For this review, take the finished solid that the model builds, in its own axes (mm). A direction names the side the tool comes from. Coordinates: 2 decimals unless noted, no trailing zeros. Loops run counter-clockwise (first coordinate to the right, second up) from the corner with the lowest first, then second, coordinate; pieces in that order, holes last. Notation, with made-up numbers: M 35.5,85.25 L 41.5,85.25 A15 ccw 41.5,98.25 Z; hole C -32.5,65 d4. An arc over 180 degrees is marked long. Write each question's results on one line, items separated by ' | '. Start each with the question number.
```python
from build123d import *

# Parameters (mm, degrees)
EXTRUDE_1_DEPTH     = 20
SKETCH_2_R          = 2
CUT_EXTRUDE_1_DEPTH = 20


with BuildPart() as part:
    # 草图1 → 凸台-拉伸1 (new body)
    with BuildSketch(Plane.XY):
        Polygon((-17.175607408, 36.360314389), (-7.175607408, 36.360314389), (2.824392592, 36.360314389), (2.824392592, 34.360314389), (-17.175607408, 34.360314389), (-17.175607408, -0.639685611), (-17.175607408, -2.639685611), (-47.175607408, -2.639685611), (-47.175607408, -0.639685611), (-19.175607408, -0.639685611), (-19.175607408, 36.360314389), align=None)
    extrude(amount=EXTRUDE_1_DEPTH)

    # 草图2 → 切除-拉伸1 (cut)
    with BuildSketch(Plane(origin=(0, 36.360314389, 0), x_dir=(1, 0, 0), z_dir=(0, 1, 0))):
        with Locations((-2.175607408, -10)):
            Circle(SKETCH_2_R)
    extrude(amount=-CUT_EXTRUDE_1_DEPTH, mode=Mode.SUBTRACT)


solid = part.part
```
Q1. For faces 4 (the face through (-19.176, 18, 10)), 5 (the face through (-7, 34.36, 10)), 6 (the face through (-8, 36.36, 10)), list the 3-axis set-ups (+Z, -Z, +X, -X, +Y, -Y) from which the entire face can be reached by the end or side of a thin tool; tool diameter is ignored.
Q2. To check wall thickness, follow line 1 along X through (y, z) = (35.65, 10); line 2 along Y through (x, z) = (-33, 15.5); line 3 along X through (y, z) = (18.5, 15). State the ranges of each line that lie inside material, in increasing order.
Q3. Take a section at B-B, the plane z = 16.5. Give the boundary of the cut face in (x, y).
Q4. Take a section at A-A, the plane z = 10. Give the boundary of the cut face in (x, y), then the cut area to 3 significant figures.
Q5. Insertion check: P1, Ø5, axis at y = 16, z = 11.5, coming from the -X side; P2, Ø5, axis at x = -26, z = 2.5, coming from the +Y side. Each pin has a flat end and moves straight along its axis. Give the tip position at first contact, or say it passes through.
Q6. Take a section at C-C, the plane y = 20. Give the boundary of the cut face in (x, z).
Q7. Take a section at D-D, the plane x = -13. Give the boundary of the cut face in (y, z), then the cut area to 3 significant figures.
Q8. The part is to be moulded in two halves that separate along X. For faces 1 (the face through (-32, -2.64, 10)), 2 (the face through (-0.268, 35.374, 9.399)), 3 (the face through (-17.176, 16, 10)), say which applies: pulls with the +X half, pulls with the -X half, needs draft (parallel to the pull), parting line crosses it, or undercut.
Results:
1) face 4: +Z, -Z, -X, +Y | face 5: +Z, -Z, +X, -Y | face 6: +Z, -Z, +X, -X, +Y
2) line 1: -19.18 to -4.18, -0.18 to 2.82 | line 2: -2.64 to -0.64 | line 3: -19.18 to -17.18
3) outline: M -47.18,-2.64 L -17.18,-2.64 L -17.18,34.36 L 2.82,34.36 L 2.82,36.36 L -19.18,36.36 L -19.18,-0.64 L -47.18,-0.64 Z
4) outline: M -47.18,-2.64 L -17.18,-2.64 L -17.18,34.36 L -4.18,34.36 L -4.18,36.36 L -19.18,36.36 L -19.18,-0.64 L -47.18,-0.64 Z; M -0.18,34.36 L 2.82,34.36 L 2.82,36.36 L -0.18,36.36 Z | area: 166 mm^2
5) P1: x = -19.18 | P2: y = -0.64
6) outline: M -19.18,0 L -17.18,0 L -17.18,20 L -19.18,20 Z
7) outline: M 34.36,0 L 36.36,0 L 36.36,20 L 34.36,20 Z | area: 40.0 mm^2
8) face 1: needs draft | face 2: undercut | face 3: pulls with the +X half
